Design review of the part built by this model. Coordinates are the model's own, in mm. A direction names the side the tool comes from. Give positions to 0.01 mm unless a question says otherwise; leave off trailing zeros. Write each loop counter-clockwise with the first axis right and the second up, starting at its lowest first coordinate (ties: lowest second). Pieces come first, ordered by that corner, then holes. Notation, with made-up numbers: M -28.5,10 L 30.5,10 A23 ccw 30.5,19 Z; hole C 43,62.5 d1. An arc over 180 degrees is marked long. Answer in a Markdown table with one row per item.
```python
from build123d import *

# Parameters (mm, degrees)
SKETCH1_W           = 62.48
SKETCH1_H           = 25.32
SKETCH1_R           = 1.5
BOSS_EXTRUDE1_DEPTH = 3
SKETCH2_W           = 1.040030553
SKETCH2_H           = 5.915173771
SKETCH2_W_2         = 4.61513558
SKETCH2_H_2         = 9.230271158
BOSS_EXTRUDE2_DEPTH = 2


with BuildPart() as part:
    # Sketch1 → Boss-Extrude1 (new body)
    with BuildSketch(Plane(origin=(0, 0, 0), x_dir=(1, 0, 0), z_dir=(0, 1, 0))):
        Rectangle(SKETCH1_W, SKETCH1_H)
        with Locations(Location((28.7, 10.16, 0), (0, 0, 270))):
            Circle(SKETCH1_R, mode=Mode.SUBTRACT)
        with Locations(Location((28.7, -10.16, 0), (0, 0, 270))):
            Circle(SKETCH1_R, mode=Mode.SUBTRACT)
        with Locations(Location((-28.7, 10.16, 0), (0, 0, 270))):
            Circle(SKETCH1_R, mode=Mode.SUBTRACT)
        with Locations(Location((-28.7, -10.16, 0), (0, 0, 270))):
            Circle(SKETCH1_R, mode=Mode.SUBTRACT)
    extrude(amount=BOSS_EXTRUDE1_DEPTH)

    # Sketch2 → Boss-Extrude2 (add)
    with BuildSketch(Plane(origin=(0, 3, 0), x_dir=(1, 0, 0), z_dir=(0, 1, 0))):
        with Locations((-18.163108198, -9.067766385)):
            Rectangle(SKETCH2_W, SKETCH2_H)
        Rectangle(SKETCH2_W_2, SKETCH2_H_2)
        with Locations((-20.703108198, -9.067766385)):
            Rectangle(SKETCH2_W, SKETCH2_H)
        with Locations((-15.623108198, -9.067766385)):
            Rectangle(SKETCH2_W, SKETCH2_H)
        with Locations((-13.083108197, -9.067766385)):
            Rectangle(SKETCH2_W, SKETCH2_H)
        with Locations((-10.543108198, -9.067766385)):
            Rectangle(SKETCH2_W, SKETCH2_H)
        with Locations((-8.003108198, -9.067766385)):
            Rectangle(SKETCH2_W, SKETCH2_H)
        with Locations((-5.463108198, -9.067766385)):
            Rectangle(SKETCH2_W, SKETCH2_H)
        with Locations((-2.923108198, -9.067766385)):
            Rectangle(SKETCH2_W, SKETCH2_H)
        with Locations((-0.383108198, -9.067766385)):
            Rectangle(SKETCH2_W, SKETCH2_H)
        with Locations((2.156891803, -9.067766385)):
            Rectangle(SKETCH2_W, SKETCH2_H)
        with Locations((4.696891802, -9.067766385)):
            Rectangle(SKETCH2_W, SKETCH2_H)
        with Locations((7.236891803, -9.067766385)):
            Rectangle(SKETCH2_W, SKETCH2_H)
        with Locations((9.776891802, -9.067766385)):
            Rectangle(SKETCH2_W, SKETCH2_H)
        with Locations((12.316891803, -9.067766385)):
            Rectangle(SKETCH2_W, SKETCH2_H)
        with Locations((14.856891803, -9.067766385)):
            Rectangle(SKETCH2_W, SKETCH2_H)
        with Locations((17.396891803, -9.067766385)):
            Rectangle(SKETCH2_W, SKETCH2_H)
        with Locations((19.936891802, -9.067766385)):
            Rectangle(SKETCH2_W, SKETCH2_H)
    extrude(amount=BOSS_EXTRUDE2_DEPTH)


solid = part.part
```
1) For faces 1 (the face through (-10.6, 4, 6.11)), 2 (the face through (-2.403, 4, 9)), 3 (the face through (20, 4, 12.025)), list the 3-axis set-ups (+Z, -Z, +X, -X, +Y, -Y) from which the entire face can be reached by the end or side of a thin tool; tool diameter is ignored.
Geometry says:
| item | result |
|---|---|
| face 1 | -Z, +X, -X, +Y |
| face 2 | +Z, -Z, +Y |
| face 3 | +Z, +X, -X, +Y |
2) Insertion check: P1, Ø10, axis at x = 13.5, z = -5, coming from the +Y side; P2, Ø0.6, axis at x = -1, y = 4, coming from the +Z side; P3, Ø1.1, axis at x = 20, y = 4.5, coming from the -Z side. Each pin has a flat end and moves straight along its axis. Give the tip position at first contact, or say it passes through.
Geometry says:
| item | result |
|---|---|
| P1 | y = 3 |
| P2 | z = 12.03 |
| P3 | z = 6.11 |
3) Add section A-A (x = 28.7). Write out the cut boundary in (y, z), and give its area (3 significant figures).
Geometry says:
| item | result |
|---|---|
| outline | M 0,-12.66 L 3,-12.66 L 3,-11.66 L 0,-11.66 Z; M 0,-8.66 L 3,-8.66 L 3,8.66 L 0,8.66 Z; M 0,11.66 L 3,11.66 L 3,12.66 L 0,12.66 Z |
| area | 58.0 mm^2 |
4) To check wall thickness, follow probe 1 along X at (y, z) = (0.85, -10.16); probe 2 along X at (y, z) = (1.9, -9.25); probe 3 along Y at (x, z) = (-3, -8.75). State the ranges of each line that lie inside material, in increasing order. Write a range as [from, to].
Geometry says:
| item | result |
|---|---|
| probe 1 | [-31.24, -30.2], [-27.2, 27.2], [30.2, 31.24] |
| probe 2 | [-31.24, -29.89], [-27.51, 27.51], [29.89, 31.24] |
| probe 3 | [0, 3] |
5) Add section C-C (y = 1.1). Write out the cut boundary in (x, z), and give its area (3 significant figures).
Geometry says:
| item | result |
|---|---|
| outline | M -31.24,-12.66 L 31.24,-12.66 L 31.24,12.66 L -31.24,12.66 Z; hole C -28.7,-10.16 d3; hole C -28.7,10.16 d3; hole C 28.7,-10.16 d3; hole C 28.7,10.16 d3 |
| area | 1,550 mm^2 |
6) Add section D-D (z = -1). Write out the cut boundary in (x, y).
Geometry says:
| item | result |
|---|---|
| outline | M -31.24,0 L 31.24,0 L 31.24,3 L 2.31,3 L 2.31,5 L -2.31,5 L -2.31,3 L -31.24,3 Z |
7) The part is to be moulded in two halves that separate along X. For faces 4 (the face through (-5.983, 4, 9)), 5 (the face through (-8.523, 4, 9)), 6 (the face through (15, 4, 6.11)), 7 (the face through (-2.308, 4, 0)), say which applies: released by +X, released by -X, zero draft, split by the parting line, or undercut.
Geometry says:
| item | result |
|---|---|
| face 4 | undercut |
| face 5 | undercut |
| face 6 | zero draft |
| face 7 | released by -X |
8) Add section B-B (z = -10.16). Write out the cut boundary in (x, y), and give its area (3 significant figures).
Geometry says:
| item | result |
|---|---|
| outline | M -31.24,0 L -30.2,0 L -30.2,3 L -31.24,3 Z; M -27.2,0 L 27.2,0 L 27.2,3 L -27.2,3 Z; M 30.2,0 L 31.24,0 L 31.24,3 L 30.2,3 Z |
| area | 169 mm^2 |
